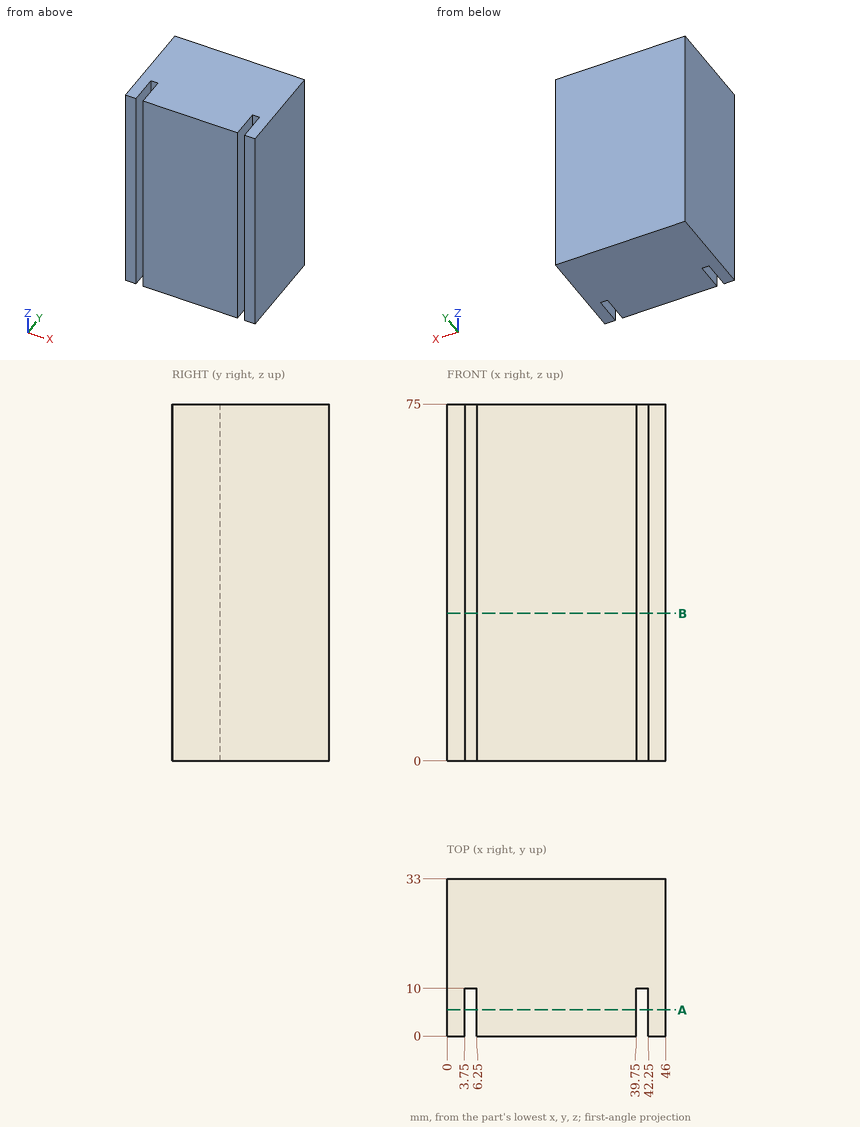
Could you check a few things on this drawing? It's one solid part, dimensions in mm from its lowest x, y, z. Round coordinates to 2 decimals unless told otherwise and drop trailing zeros. Order: outer loops, then holes, each group sorted by start corner. A loop starts at its lowest first (then second) coordinate and runs counter-clockwise, first axis right, second up. Notation, with made-up numbers: M 11.25,4.5 L 38.25,4.5 A23 cw 38.25,30.5 Z; hole C 80,56 d2. An arc over 180 degrees is marked long. One line per item, written item: value.
(1) Imagine slicing it at A-A (y = 5.5). Write out the boundary of the cut face in (x, z), and give its area (4 significant figures).
Ans:
outline: M 0,0 L 3.75,0 L 3.75,75 L 0,75 Z; M 6.25,0 L 39.75,0 L 39.75,75 L 6.25,75 Z; M 42.25,0 L 46,0 L 46,75 L 42.25,75 Z
area: 3,075 mm^2
(2) I need wall thicknesses on line 1 along X through (y, z) = (7, 5); line 2 along Y through (x, z) = (41.5, 8.5). Which ranges of each line are inside material? Lowest first, please. Write a range as from..to.
Ans:
line 1: x = 0..3.75, 6.25..39.75, 42.25..46
line 2: y = 10..33
(3) I'm going to push a flat-ended pin straight in: P1, Ø0.8, axis at x = 40.5, z = 45.5, coming from the -Y side. Where does the tip first touch, or does it pass through?
Ans:
P1: stops at y = 10
(4) Imagine slicing it at B-B (z = 31). Write out the boundary of the cut face in (x, y).
Ans:
outline: M 0,0 L 3.75,0 L 3.75,10 L 6.25,10 L 6.25,0 L 39.75,0 L 39.75,10 L 42.25,10 L 42.25,0 L 46,0 L 46,33 L 0,33 Z
